Autodesk Inventor part; units mm, degrees
ref_plane "YZ Plane" through (0, 0, 0) normal (1, 0, 0) x (0, 1, 0)
ref_plane "XZ Plane" through (0, 0, 0) normal (0, 1, 0) x (-1, 0, 0)
ref_plane "XY Plane" through (0, 0, 0) normal (0, 0, 1) x (1, 0, 0)
sketch "Sketch2" plane through (0, 0, 0) normal (0, 1, 0) x (-1, 0, 0)
  line L0 (-2.3812, 0) -> (-26.1937, 0) construction
  line L1 (-28.575, -2.3812) -> (-28.575, -26.1937) construction
  line L2 (-26.1937, -28.575) -> (-2.3812, -28.575) construction
  line L3 (0, -26.1937) -> (0, -2.3812) construction
  line L4 (-27.8023, -27.8024) -> (0.7727, 0.7726) construction
  line L5 (0, -28.575) -> (-28.575, 0) construction
  circle A0 centre (-14.2875, -14.2875) radius 6.35 construction
  line L6 (-14.2875, -28.575) -> (-14.2875, 0) construction
  line L7 (0, -14.2875) -> (-28.575, -14.2875) construction
  arc A1 (-2.3812, -28.575) -> (0, -26.1937) centre (-2.3812, -26.1937) ccw
  line L8 (0, -26.1937) -> (-7.0569, -15.6084)
  line L9 (-2.3812, -28.575) -> (-12.9666, -21.5181)
  arc A2 (-28.575, -26.1937) -> (-26.1937, -28.575) centre (-26.1937, -26.1937) ccw
  arc A3 (-26.1937, 0) -> (-28.575, -2.3812) centre (-26.1937, -2.3813) ccw
  arc A4 (0, -2.3812) -> (-2.3812, 0) centre (-2.3812, -2.3812) ccw
  line L10 (-15.6084, -21.5181) -> (-26.1937, -28.575)
  line L11 (-28.575, -26.1937) -> (-21.5181, -15.6084)
  line L12 (-21.5181, -12.9666) -> (-28.575, -2.3812)
  line L13 (-26.1937, 0) -> (-15.6084, -7.0569)
  line L14 (-12.9666, -7.0569) -> (-2.3812, 0)
  line L15 (0, -2.3812) -> (-7.0569, -12.9666)
  arc A5 (-12.9666, -21.5181) -> (-15.6084, -21.5181) centre (-14.2875, -23.4994) ccw
  arc A6 (-7.0569, -12.9666) -> (-7.0569, -15.6084) centre (-5.0756, -14.2875) ccw
  arc A7 (-15.6084, -7.0569) -> (-12.9666, -7.0569) centre (-14.2875, -5.0756) ccw
  arc A8 (-21.5181, -15.6084) -> (-21.5181, -12.9666) centre (-23.4994, -14.2875) ccw
  circle A9 centre (-26.0719, -26.072) radius 0.7938
  circle A10 centre (-14.2875, -14.2875) radius 16.6688 construction
  circle A11 centre (-23.8268, -23.8269) radius 0.7938
  circle A12 centre (-21.5818, -21.5819) radius 0.7938
  circle A13 centre (-19.3367, -19.3368) radius 0.7938
  circle A14 centre (-2.503, -26.0719) radius 0.7938
  circle A15 centre (-4.7481, -23.8268) radius 0.7938
  circle A16 centre (-6.9931, -21.5818) radius 0.7938
  circle A17 centre (-9.2382, -19.3367) radius 0.7938
  circle A18 centre (-2.5031, -2.503) radius 0.7938
  circle A19 centre (-4.7482, -4.7481) radius 0.7938
  circle A20 centre (-6.9932, -6.9931) radius 0.7938
  circle A21 centre (-9.2383, -9.2382) radius 0.7938
  circle A22 centre (-26.072, -2.5031) radius 0.7938
  circle A23 centre (-23.8269, -4.7482) radius 0.7938
  circle A24 centre (-21.5819, -6.9932) radius 0.7938
  circle A25 centre (-19.3368, -9.2383) radius 0.7938
  point P0 (0, 0)
  point P1 (-7.9375, -14.2875)
  point P2 (-14.2875, -20.6375)
  point P3 (-20.6375, -14.2875)
  point P4 (-14.2875, -7.9375)
  dimension "d0" = 27.813
  dimension "d1" = 27.8131
  dimension "d2" = 12.7
  dimension "d3" = 2.3813
  dimension "d4" = 2.3813
  dimension "d5" = 2.3813
  dimension "d6" = 1.5875
  dimension "d7" = 33.3375
  dimension "d10" = 3.175
  dimension "d17" = 360
extrude "Extrusion1" add sketch "Sketch2" along normal blind 1.5875
sketch "Sketch3" plane through (0, 0, 0) normal (0, -1, 0) x (1, 0, 0)
  circle A0 centre (14.2875, -14.2875) radius 3.9688
  circle A1 centre (14.2875, -14.2875) radius 1.5875
  point P0 (0, 0)
  dimension "d21" = 7.9375
  dimension "d22" = 3.175
extrude "Extrusion2" add sketch "Sketch3" along normal blind 3.175
extrude "Extrusion3" cut sketch "Sketch3" against normal through all contours A1
fillet "Fillet1" radius 1.5875 1 edges at (10.3187, 0, -14.2875)
properties part number "servoHornX"
Could you check a few things on this model? Use its own coordinates, in mm. A direction names the side the tool comes from. Round coordinates to 2 decimals unless told otherwise and drop trailing zeros. Order: outer loops, then holes, each group sorted by start corner. A loop starts at its lowest first (then second) coordinate and runs counter-clockwise, first axis right, second up.
(1) Imagine slicing it at C-C (y = -1.25). Write out the boundary of the cut face in (x, z) (1 decimal).
Response values:
outline: circle Ø8 at (14.3, -14.3); hole circle Ø3.2 at (14.3, -14.3)
(2) Imagine slicing it at A-A (y = 1.2). Count the separate pieces of the cut face and the enclosed holes in it, plus the area to 3 significant figures.
Response values:
separate pieces: 1
enclosed holes: 17
area: 396 mm2
(3) Which directions (+Z, -Z, +X, -X, +Y, -Y) give clear straight access to the entire face, cutting with the end or side of a thin tool? Please do faces 1 (the flat face through (3.48, 0.78, -7.6)), 2 (the flat face through (7.75, 0.78, -3.58)), 3 (the cylindrical face through (13.427, -2.37, -10.413)).
Response values:
face 1: -X, +Y, -Y
face 2: +Z, +Y, -Y
face 3: -Y
(4) Please list where these lines run through material, in increasing order: line 1 along Z through (x, y) = (8.75, 0.5); line 2 along Y through (x, z) = (12.25, -21.25); line 3 along X through (y, z) = (0.1, -4.75).
Response values:
line 1: z = -24.33 to -19.96, -18.71 to -9.86, -8.61 to -4.25
line 2: y = 0 to 1.59
line 3: x = 1.58 to 3.95, 5.54 to 9.51, 19.07 to 23.03, 24.62 to 27
(5) If we mould it in two halves opening along X, with no side actions, what happens to faces 4 (the flat face through (11, 1.588, -14)), 5 (the cylindrical face through (18.604, 0.783, -8.934)), 6 (the flat face through (25.1, 0.78, -20.98))? For each: released by +X, released by -X, zero draft, split by the parting line, or undercut.
Response values:
face 4: zero draft
face 5: undercut
face 6: released by +X
